from build123d import *

# Parameters (mm, degrees)
F1_DEPTH  = 45
F3_DEPTH  = 10
F4_R      = 2
F5_R      = 3.2
F6_DEPTH  = 10
F2_W      = 14.6
F2_H      = 37.61
F7_DEPTH  = 10
F8_R      = 3
F9_R      = 1.99999
F2_W_2    = 6.8
F2_H_2    = 0.6
F10_DEPTH = 0.6


# Not quite as in the source:
# - a fillet or chamfer is up to 0.001 mm smaller than in the source, because OpenCascade refuses the exact size
# - a feature names something its author has since deleted; it is built from what else it names


with BuildPart() as f1:
    # F0 (on Right) → F1 (new body)
    with BuildSketch(Plane.YZ):
        Polygon((37.61, 0), (0, 0), (0, 67.3), (-10, 67.3), (-10, -10), (37.61, -10), align=None)
    extrude(amount=F1_DEPTH)

    # F2 (on face) → F3 (cut)
    with BuildSketch(Plane.XY):
        with BuildLine():
            Line((13.2, 6.11), (13.2, 31.11))
            ThreePointArc((13.2, 31.11), (10, 34.31), (6.8, 31.11))
            Line((6.8, 31.11), (6.8, 23.91))
            Line((6.8, 23.91), (6.8, 23.31))
            Line((6.8, 23.31), (6.8, 11.41))
            Line((6.8, 11.41), (6.8, 10.81))
            Line((6.8, 10.81), (6.8, 6.11))
            ThreePointArc((6.8, 6.11), (10, 2.91), (13.2, 6.11))
        make_face()
        with BuildLine():
            Line((38.2, 23.31), (38.2, 23.91))
            Line((38.2, 23.91), (38.2, 31.11))
            ThreePointArc((38.2, 31.11), (35, 34.31), (31.8, 31.11))
            Line((31.8, 31.11), (31.8, 6.11))
            ThreePointArc((31.8, 6.11), (35, 2.91), (38.2, 6.11))
            Line((38.2, 6.11), (38.2, 10.81))
            Line((38.2, 10.81), (38.2, 11.41))
            Line((38.2, 11.41), (38.2, 23.31))
        make_face()
    extrude(amount=-F3_DEPTH, mode=Mode.SUBTRACT)

    # F4
    f4_edges = [f1.edges().sort_by_distance(p)[0] for p in [
        (22.5, 37.61, -10),
        (22.5, -10, -10),
        (22.5, 0, 67.3),
        (22.5, -10, 67.3),
    ]]
    fillet(f4_edges, radius=F4_R)

    # F5 (on face) → F6 (cut)
    with BuildSketch(Plane.XZ.offset(10)):
        with Locations((10, 58.8)):
            Circle(F5_R)
        with Locations((22.5, 58.8)):
            Circle(F5_R)
        with Locations((35, 58.8)):
            Circle(F5_R)
        with Locations((35, 46.3)):
            Circle(F5_R)
        with Locations((22.5, 46.3)):
            Circle(F5_R)
        with Locations((10, 46.3)):
            Circle(F5_R)
        with Locations((10, 33.8)):
            Circle(F5_R)
        with Locations((22.5, 33.8)):
            Circle(F5_R)
        with Locations((35, 33.8)):
            Circle(F5_R)
    extrude(amount=-F6_DEPTH, mode=Mode.SUBTRACT)

    # F2 (on face) → F7 (cut)
    with BuildSketch(Plane.XY):
        with Locations((22.5, 18.805)):
            Rectangle(F2_W, F2_H)
    extrude(amount=-F7_DEPTH, mode=Mode.SUBTRACT)

    # F8
    f8_edges = [f1.edges().sort_by_distance(p)[0] for p in [
        (29.8, 0, -5),
        (15.2, 0, -5),
    ]]
    fillet(f8_edges, radius=F8_R)

    # F9 (radius 2 in the source; OpenCascade refuses exactly that, so slightly less here)
    f9_edges = [f1.edges().sort_by_distance(p)[0] for p in [
        (15.2, 37.61, -4),
        (15.2, 37.024214, -9.414214),
        (37.4, 37.61, 0),
        (7.6, 37.61, 0),
    ]]
    fillet(f9_edges, radius=F9_R)

    # F2 (on face) → F10 (cut)
    with BuildSketch(Plane.XY):
        with Locations((3.4, 11.11)):
            Rectangle(F2_W_2, F2_H_2)
        with Locations((3.4, 23.61)):
            Rectangle(F2_W_2, F2_H_2)
        with Locations((41.6, 11.11)):
            Rectangle(F2_W_2, F2_H_2)
        with Locations((41.6, 23.61)):
            Rectangle(F2_W_2, F2_H_2)
    extrude(amount=-F10_DEPTH, mode=Mode.SUBTRACT)


solid = f1.part
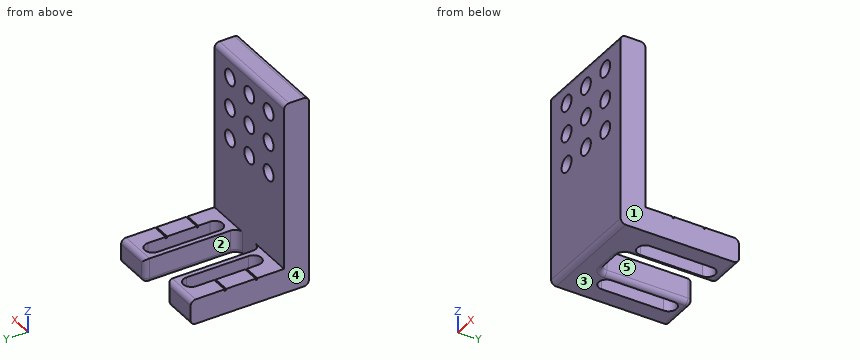
Verification items for the finished model (mm, model axes). Face numbers are marked on the shaded views. A direction names the side the tool comes from. Coordinates: 2 decimals unless noted, no trailing zeros. Order: outer loops, then holes, each group sorted by start corner. A loop starts at its lowest first (then second) coordinate and runs counter-clockwise, first axis right, second up. Notation, with made-up numbers: M -27,-18.75 L 16,-18.75 A11 ccw 16,-8.75 Z; hole C -24,10.25 d9. An arc over 180 degrees is marked long. Return JSON: item names as keys, results as strings.
1) Cross-section at D-D, the plane x = 5. Record the boundary of the cut face in (y, z).
Answer list:
{"outline": "M -10,-8 A2 ccw -8,-10 L 35.61,-10 A2 ccw 37.61,-8 L 37.61,-2 A2 ccw 35.61,0 L 23.91,0 L 23.91,-0.6 L 23.31,-0.6 L 23.31,0 L 11.41,0 L 11.41,-0.6 L 10.81,-0.6 L 10.81,0 L 0,0 L 0,65.3 A2 ccw -2,67.3 L -8,67.3 A2 ccw -10,65.3 Z"}
2) Cross-section at A-A, the plane x = 35. Record the boundary of the cut face in (y, z).
Answer list:
{"outline": "M -10,-8 A2 ccw -8,-10 L 2.91,-10 L 2.91,0 L 0,0 L 0,30.6 L -10,30.6 Z; M -10,37 L 0,37 L 0,43.1 L -10,43.1 Z; M -10,49.5 L 0,49.5 L 0,55.6 L -10,55.6 Z; M -10,62 L 0,62 L 0,65.3 A2 ccw -2,67.3 L -8,67.3 A2 ccw -10,65.3 Z; M 34.31,-10 L 35.61,-10 A2 ccw 37.61,-8 L 37.61,-2 A2 ccw 35.61,0 L 34.31,0 Z"}
3) Release check for a two-part mould opening along X. For the marked faces 1, 2 and 3 record: +X half, -X half, draft (parallel to the pull), parting line (faces both ways), or undercut.
Answer list:
{"face 1": "+X half", "face 2": "undercut", "face 3": "draft"}
4) Cross-section at C-C, the plane y = 15. Count the separate pieces of the cut face and the enclosed holes in it, and give its area (3 significant figures).
Answer list:
{"separate pieces": "4", "enclosed holes": "0", "area": "174 mm2"}
5) Access from +Z, -Z, +X, -X, +Y, -Y to the whole of each face (thin tool, end or side, straight path). Record for the marked faces 4 and 5.
Answer list:
{"face 4": "+Z, -Z, -X, +Y, -Y", "face 5": "+Z, -Z, +Y"}
6) Cross-section at B-B, the plane z = 46.3. Record the boundary of the cut face in (x, y).
Answer list:
{"outline": "M 0,-10 L 6.8,-10 L 6.8,0 L 0,0 Z; M 13.2,-10 L 19.3,-10 L 19.3,0 L 13.2,0 Z; M 25.7,-10 L 31.8,-10 L 31.8,0 L 25.7,0 Z; M 38.2,-10 L 45,-10 L 45,0 L 38.2,0 Z"}
7) Gauge pin test, flat ends, axial feed: pin 1 (10 mm diameter, centred on x = 15, z = 41, fed in from +Y); pin 2 (3 mm diameter, centred on y = 27, z = 3, fed in from +X) (3 decimals); pin 3 (0.7 mm diameter, centred on x = 40.5, z = -0.5, fed in from +Y); pin 4 (3 mm diameter, centred on x = 15, y = 3.5, fed in from -Z). Record the tip position at first contact, or that the pin passes through.
Answer list:
{"pin 1": "y = 0", "pin 2": "through", "pin 3": "y = 37.25", "pin 4": "z = -9.98"}
8) Thickness scan on L1, parallel to Z at x = 10, y = -7; L2, parallel to X at y = -3.5, z = 44; L3, parallel to Y at x = 21, z = -2. Record the ranges inside material, lowest first. Write a range as [from, to].
Answer list:
{"L1": "[-10, 30.6], [37, 43.1], [49.5, 55.6], [62, 67.3]", "L2": "[0, 7.78], [12.22, 20.28], [24.72, 32.78], [37.22, 45]", "L3": "[-10, 0]"}
